Read the model definition and answer for the solid it produces. Units are mm, in the model's axes. A direction names the side the tool comes from. Round coordinates to 2 decimals unless told otherwise and drop trailing zeros. Write each loop counter-clockwise with the first axis right and the second up, starting at its lowest first coordinate (ties: lowest second). Pieces come first, ordered by that corner, then holes.
from build123d import *

# Parameters (mm, degrees)
SKETCH1_R           = 2.5527
SKETCH1_R_2         = 1.8288
SKETCH1_R_3         = 2.0193
BOSS_EXTRUDE1_DEPTH = 2.286
CUT_EXTRUDE1_DEPTH  = 128.490937977
FILLET1_R           = 1.5875


with BuildPart() as part:
    # Sketch1 → Boss-Extrude1 (new body)
    with BuildSketch(Plane.XY.offset(1.5875)):
        with BuildLine():
            Line((18.288, -65.0875), (18.288, -24.13))
            ThreePointArc((18.288, -24.13), (19.775897552, -20.537897552), (23.368, -19.05))
            Line((23.368, -19.05), (90.678, -19.05))
            ThreePointArc((90.678, -19.05), (94.270102448, -17.562102448), (95.758, -13.97))
            Line((95.758, -13.97), (95.758, 24.13))
            ThreePointArc((95.758, 24.13), (94.270102448, 27.722102448), (90.678, 29.21))
            Line((90.678, 29.21), (23.368, 29.21))
            ThreePointArc((23.368, 29.21), (19.775897552, 30.697897552), (18.288, 34.29))
            Line((18.288, 34.29), (18.288, 77.7875))
            ThreePointArc((18.288, 77.7875), (16.428128061, 82.277628061), (11.938, 84.1375))
            Line((11.938, 84.1375), (-11.938, 84.1375))
            ThreePointArc((-11.938, 84.1375), (-16.428128061, 82.277628061), (-18.288, 77.7875))
            Line((-18.288, 77.7875), (-18.288, -65.0875))
            ThreePointArc((-18.288, -65.0875), (-16.428128061, -69.577628061), (-11.938, -71.4375))
            Line((-11.938, -71.4375), (11.938, -71.4375))
            ThreePointArc((11.938, -71.4375), (16.428128061, -69.577628061), (18.288, -65.0875))
        make_face()
        with Locations(Location((87.376, 18.415, 0), (0, 0, 180))):
            Circle(SKETCH1_R, mode=Mode.SUBTRACT)
        with Locations(Location((30.734, -8.255, 0), (0, 0, 180))):
            Circle(SKETCH1_R, mode=Mode.SUBTRACT)
        with Locations(Location((0, -13.0175, 0), (0, 0, 180))):
            Circle(SKETCH1_R_2, mode=Mode.SUBTRACT)
        with Locations(Location((0, 6.0325, 0), (0, 0, 180))):
            Circle(SKETCH1_R_2, mode=Mode.SUBTRACT)
        with Locations(Location((0, 36.5125, 0), (0, 0, 180))):
            Circle(SKETCH1_R_3, mode=Mode.SUBTRACT)
        with Locations(Location((0, 55.5625, 0), (0, 0, 180))):
            Circle(SKETCH1_R_3, mode=Mode.SUBTRACT)
        with Locations(Location((12.7, -60.325, 0), (0, 0, 180))):
            Circle(SKETCH1_R, mode=Mode.SUBTRACT)
        with Locations(Location((-12.7, -60.325, 0), (0, 0, 180))):
            Circle(SKETCH1_R, mode=Mode.SUBTRACT)
        with Locations(Location((0, -34.925, 0), (0, 0, 180))):
            Circle(SKETCH1_R, mode=Mode.SUBTRACT)
    extrude(amount=-BOSS_EXTRUDE1_DEPTH)

    # Sketch2 → Cut-Extrude1 (cut, through all)
    with BuildSketch(Plane.XY.offset(1.5875)):
        Polygon((79.922815554, 18.415), (38.187184446, 18.415), (59.055, 8.589346937), align=None)
        Polygon((51.601815554, 5.08), (30.734, 14.905653063), (30.734, -4.745653063), align=None)
        Polygon((79.922815554, -8.255), (59.055, 1.570653063), (38.187184446, -8.255), align=None)
        Polygon((87.376, 14.905653063), (66.508184446, 5.08), (87.376, -4.745653063), align=None)
    extrude(amount=-CUT_EXTRUDE1_DEPTH, mode=Mode.SUBTRACT)

    # Fillet1
    fillet1_edges = [part.edges().sort_by_distance(p)[0] for p in [
        (30.734, 14.905653063, 0.4445),
        (51.601815554, 5.08, 0.4445),
        (59.055, 1.570653063, 0.4445),
        (79.922815554, -8.255, 0.4445),
        (38.187184446, -8.255, 0.4445),
        (66.508184446, 5.08, 0.4445),
        (87.376, 14.905653063, 0.4445),
        (87.376, -4.745653063, 0.4445),
        (38.187184446, 18.415, 0.4445),
        (79.922815554, 18.415, 0.4445),
        (59.055, 8.589346937, 0.4445),
        (30.734, -4.745653063, 0.4445),
    ]]
    fillet(fillet1_edges, radius=FILLET1_R)


solid = part.part
Q1. Section B-B (x = 37) is taken. Determine the outline of the cut face in (y, z), then the cut area to 3 significant figures.
Verdict:
outline: (-19.05, -0.7) - (-1.8, -0.7) - (-1.8, 1.59) - (-19.05, 1.59) - close; (11.96, -0.7) - (29.21, -0.7) - (29.21, 1.59) - (11.96, 1.59) - close
area: 78.9 mm2
Q2. Which of the six approach directions +Z, -Z, +X, -X, +Y, -Y give full straight-line access (tool end or side, diameter ignored) to faces 4 (the flat face through (40.88, 10.13, 0.46)), 5 (the cylindrical face through (16.378, -69.627, 0.461))?
Verdict:
face 4: +Z, -Z
face 5: +Z, -Z, +X, -Y
Q3. Straight lines are drawn through the part: probe 1 along Y at (x, z) = (0, 1.05); probe 2 along X at (y, z) = (-7.5, 0.8); probe 3 along X at (y, z) = (75.5, 1.1). For each, find the intervals that lie inside material, in ascending order.
Verdict:
probe 1: y = -71.44 to -37.48, -32.37 to -14.85, -11.19 to 4.2, 7.86 to 34.49, 38.53 to 53.54, 57.58 to 84.14
probe 2: x = -18.29 to 28.3, 33.17 to 43.93, 74.18 to 95.76
probe 3: x = -18.29 to 18.29
Q4. Flat-ended cylindrical pins translate along their axes: pin 1 Ø3 at (x, y) = (30.734, -8.255) entering from +Z; pin 2 Ø0.7 at (x, z) = (66, 1) entering from +Y; pin 3 Ø4.5 at (x, y) = (0, 55.56) entering from -Z; pin 4 Ø0.7 at (x, z) = (64, 1) entering from -Y. Find the tip coordinate at first contact, or state that the pin passes through.
Verdict:
pin 1: passes through
pin 2: stops at y = 29.21
pin 3: stops at z = -0.7
pin 4: stops at y = -19.05
Q5. Section C-C (z = -0.1) is taken. State how many separate pieces and enclosed holes the cut face has, then the cut area to 3 significant figures.
Verdict:
separate pieces: 1
enclosed holes: 13
area: 8,470 mm2
Q6. Section D-D (y = -56) is taken. Determine the outline of the cut face in (x, z), then the cut area to 3 significant figures.
Verdict:
outline: (-18.29, -0.7) - (18.29, -0.7) - (18.29, 1.59) - (-18.29, 1.59) - close
area: 83.6 mm2
Q7. Section A-A (x = 0) is taken. Determine the outline of the cut face in (y, z).
Verdict:
outline: (-71.44, -0.7) - (-37.48, -0.7) - (-37.48, 1.59) - (-71.44, 1.59) - close; (-32.37, -0.7) - (-14.85, -0.7) - (-14.85, 1.59) - (-32.37, 1.59) - close; (-11.19, -0.7) - (4.2, -0.7) - (4.2, 1.59) - (-11.19, 1.59) - close; (7.86, -0.7) - (34.49, -0.7) - (34.49, 1.59) - (7.86, 1.59) - close; (38.53, -0.7) - (53.54, -0.7) - (53.54, 1.59) - (38.53, 1.59) - close; (57.58, -0.7) - (84.14, -0.7) - (84.14, 1.59) - (57.58, 1.59) - close
Q8. Determine the mould class of faces 1 (the cylindrical face through (-16.477, -69.528, 0.461)), 2 (the cylindrical face through (19.816, 30.659, 0.461)), 3 (the flat face through (40.666, -0.069, 0.461)) for opening direction X: pulls with the +X half, pulls with the -X half, needs draft (parallel to the pull), parting line crosses it, or undercut.
Verdict:
face 1: pulls with the -X half
face 2: pulls with the +X half
face 3: undercut
